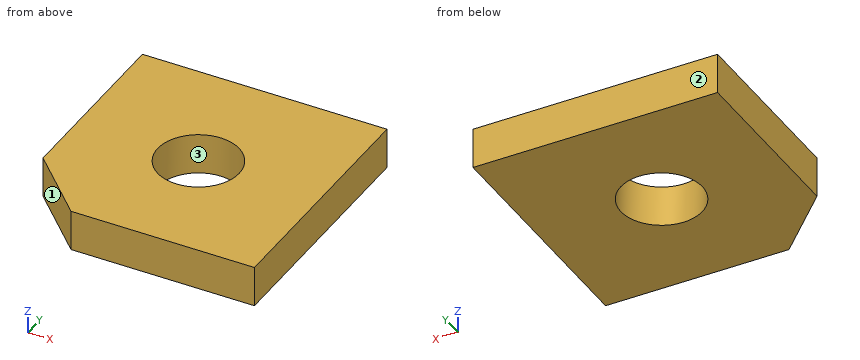
```python
from build123d import *

# Parameters (mm, degrees)
SKETCH1_W           = 76.2
SKETCH1_H           = 76.2
SKETCH1_R           = 12.7
BOSS_EXTRUDE1_DEPTH = 12.7
CHAMFER1_SIZE       = 19.05


with BuildPart() as part:
    # Sketch1 → Boss-Extrude1 (new body)
    with BuildSketch(Plane.XY):
        with Locations((-38.1, 38.1)):
            Rectangle(SKETCH1_W, SKETCH1_H)
        with Locations((-38.1, 38.1)):
            Circle(SKETCH1_R, mode=Mode.SUBTRACT)
    extrude(amount=BOSS_EXTRUDE1_DEPTH)

    # Chamfer1
    chamfer1_edges = [part.edges().sort_by_distance(p)[0] for p in [
        (-76.2, 0, 6.35),
    ]]
    chamfer(chamfer1_edges, length=CHAMFER1_SIZE)


solid = part.part
```
Geometry: final body of the model. Coordinates: model frame, mm. Face numbers are marked on the shaded views. Coordinates: 2 decimals unless noted, no trailing zeros. Order: outer loops, then holes, each group sorted by start corner. A loop starts at its lowest first (then second) coordinate and runs counter-clockwise, first axis right, second up. Notation, with made-up numbers: (52, 79.25) -> (82, 79.25) arc R18 ccw to (82, 111.25) -> close; hole circle Ø11 at (18, 46.5). An arc over 180 degrees is marked (long way). Use CSV: the item, a comma, the result in double quotes.
1) Section A-A on x = -38.1. Output: boundary loops of the cut face in (y, z), then the cut area to 3 significant figures.
Findings:
outline,"(0, 0) -> (25.4, 0) -> (25.4, 12.7) -> (0, 12.7) -> close; (50.8, 0) -> (76.2, 0) -> (76.2, 12.7) -> (50.8, 12.7) -> close"
area,"645 mm^2"
2) Line query: line 1 (Y direction, x = -38.1, z = 7.25); line 2 (Y direction, x = -31.5, z = 1.75); line 3 (Y direction, x = -66, z = 8). Output: solid intervals per line, ascending.
Findings:
line 1,"y = 0 to 25.4, 50.8 to 76.2"
line 2,"y = 0 to 27.25, 48.95 to 76.2"
line 3,"y = 8.85 to 76.2"
3) Section B-B on y = 38.1. Output: boundary loops of the cut face in (x, z).
Findings:
outline,"(-76.2, 0) -> (-50.8, 0) -> (-50.8, 12.7) -> (-76.2, 12.7) -> close; (-25.4, 0) -> (0, 0) -> (0, 12.7) -> (-25.4, 12.7) -> close"
4) Mould query, pull axis X, two halves, no side actions, for the marked faces 1, 2 and 3. Classes: +X half, -X half, draft (parallel to the pull), parting line (faces both ways), or undercut.
Findings:
face 1,"-X half"
face 2,"draft"
face 3,"undercut"
5) Section D-D on x = -66.5. Output: boundary loops of the cut face in (y, z), then the cut area to 3 significant figures.
Findings:
outline,"(9.35, 0) -> (76.2, 0) -> (76.2, 12.7) -> (9.35, 12.7) -> close"
area,"849 mm^2"
6) Section C-C on z = 10. Output: boundary loops of the cut face in (x, y).
Findings:
outline,"(-76.2, 19.05) -> (-57.15, 0) -> (0, 0) -> (0, 76.2) -> (-76.2, 76.2) -> close; hole circle Ø25.4 at (-38.1, 38.1)"
